Geometry: see drawing. Coordinates: mm, zero at the bounding-box minimum. Give positions to 0.01 mm unless a question says otherwise; leave off trailing zeros. Order: outer loops, then holes, each group sorted by start corner. A loop starts at its lowest first (then second) coordinate and runs counter-clockwise, first axis right, second up. Notation, with made-up numbers: (89.5, -6.5) - (143.5, -6.5) arc R19 cw to (143.5, 21.5) - close; hole circle Ø2 at (-31.5, -34.75). An arc over 180 degrees is marked (long way). Put each result on its own line as item: value. Start each with the question number.
1. Ray query, line 1 along Y through (x, z) = (6.25, 14); line 2 along Y through (x, z) = (4, 18); line 3 along X through (y, z) = (13.25, 27.5). Return the intervals inside material, ascending. Write a range as from..to.
2. First-contact query: P1, Ø8, axis at x = 7, y = 11.5, coming from the -Z side; P2, Ø1, axis at x = 9.5, z = 19.5, coming from the -Y side; P3, Ø8, axis at x = 13, y = 10, coming from the +Z side (1 decimal); P4, Ø8, axis at y = 12, z = 33, coming from the -X side. Flat tips, straight axial feed; report the tip coordinate or a pass-through.
3. Section B-B on y = 12.5. Return the cut outline in (x, z), plus the area to 3 significant figures.
4. Section C-C on z = 8.5. Return the cut outline in (x, y) (1 decimal), plus the area to 3 significant figures.
5. Section D-D on z = 31. Return the cut outline in (x, y) (1 decimal), plus the area to 3 significant figures.
6. Section A-A on x = 8.25. Return the cut outline in (y, z).
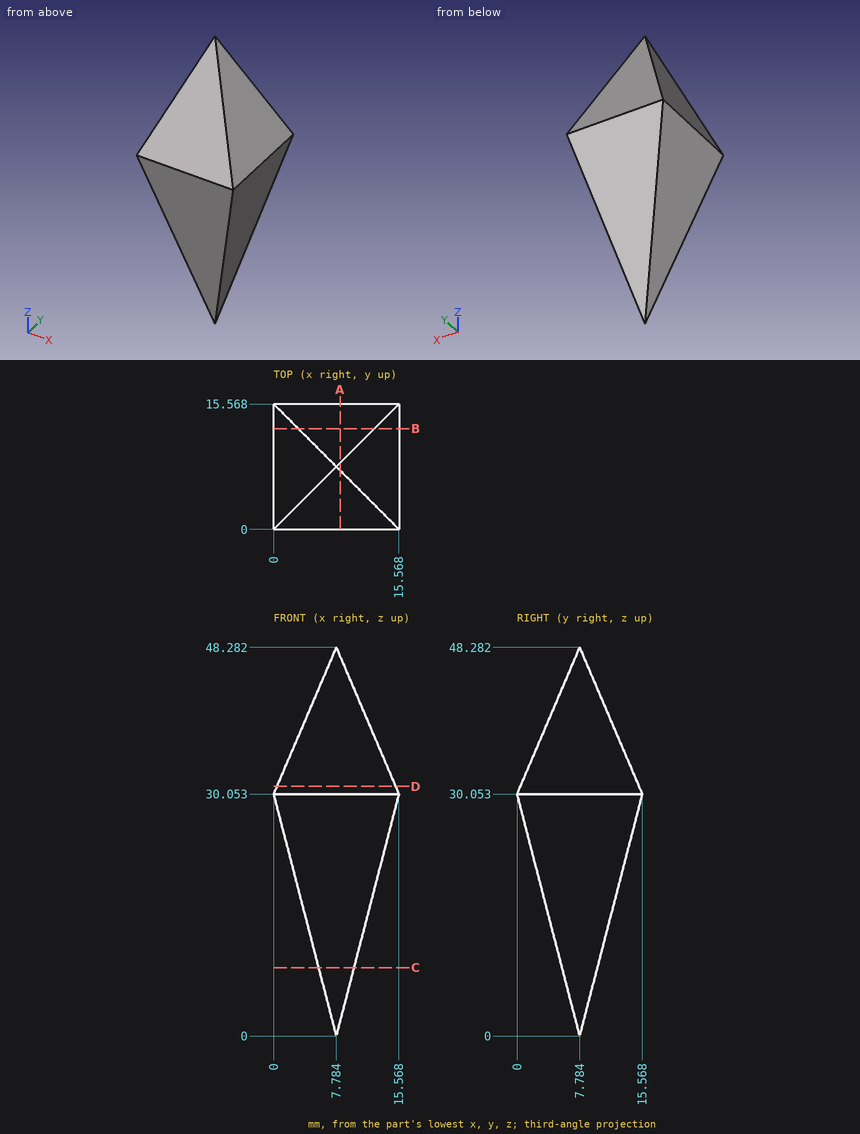
Resolved:
1. line 1: 4.16..11.41
1. line 2: 3.12..12.45
1. line 3: 0.66..14.91
2. P1: z = 0
2. P2: y = 2.6
2. P3: z = 45.2
2. P4: x = 0
3. outline: (0, 30.05) - (3.07, 18.21) - (12.5, 18.21) - (15.57, 30.05) - (12.5, 37.24) - (3.07, 37.24) - close
3. area: 238 mm^2
4. outline: (5.6, 5.6) - (10, 5.6) - (10, 10) - (5.6, 10) - close
4. area: 19.4 mm^2
5. outline: (0.4, 0.4) - (15.2, 0.4) - (15.2, 15.2) - (0.4, 15.2) - close
5. area: 218 mm^2
6. outline: (0, 30.05) - (7.32, 1.8) - (8.25, 1.8) - (15.57, 30.05) - (8.25, 47.19) - (7.32, 47.19) - close
